Job drawing, mm, ordinate dimensions from the low corner. One solid piece. A direction names the side the tool comes from. Coordinates: 2 decimals unless noted, no trailing zeros. Write each loop counter-clockwise with the first axis right and the second up, starting at its lowest first coordinate (ties: lowest second). Pieces come first, ordered by that corner, then holes. Notation, with made-up numbers: (74.25, -38) - (103.25, -38) arc R19 ccw to (103.25, -22) - close; hole circle Ø10 at (46.25, 12.25). An arc over 180 degrees is marked (long way). Put each result on its own line as item: value. Start each with the question number.
1. Saw through at D-D, the plane y = 132.1. Write the cut outline in (x, z).
2. Which spindle directions (+Z, -Z, +X, -X, +Y, -Y) get a long thin tool onto all of the face, cutting with end or side? Do the marked faces 1 and 2. Say none if no direction does.
3. Drop flat-ended pins along their axis: P1, Ø3.5, axis at x = 8, y = 7.5, coming from the +Z side; P2, Ø1.2, axis at x = 133, y = 132, coming from the +Z side. Give the stop position or say it passes through.
4. Saw through at A-A, the plane x = 74. Write the cut outline in (y, z), plus the area to 3 significant figures.
5. Saw through at C-C, the plane z = 9. Write the cut outline in (x, y), plus the area to 3 significant figures.
6. Drill centre lines: L1, parallel to Y at x = 72.5, z = 8; L2, parallel to Y at x = 7.9, z = 17.75. Where is each one in solid material? Low to high. Write a range as from..to.
7. Pull direction X, two halves, no side cores. Call the marked faces 3, 4 and 5: released by +X, released by -X, zero draft, split by the parting line, or undercut.
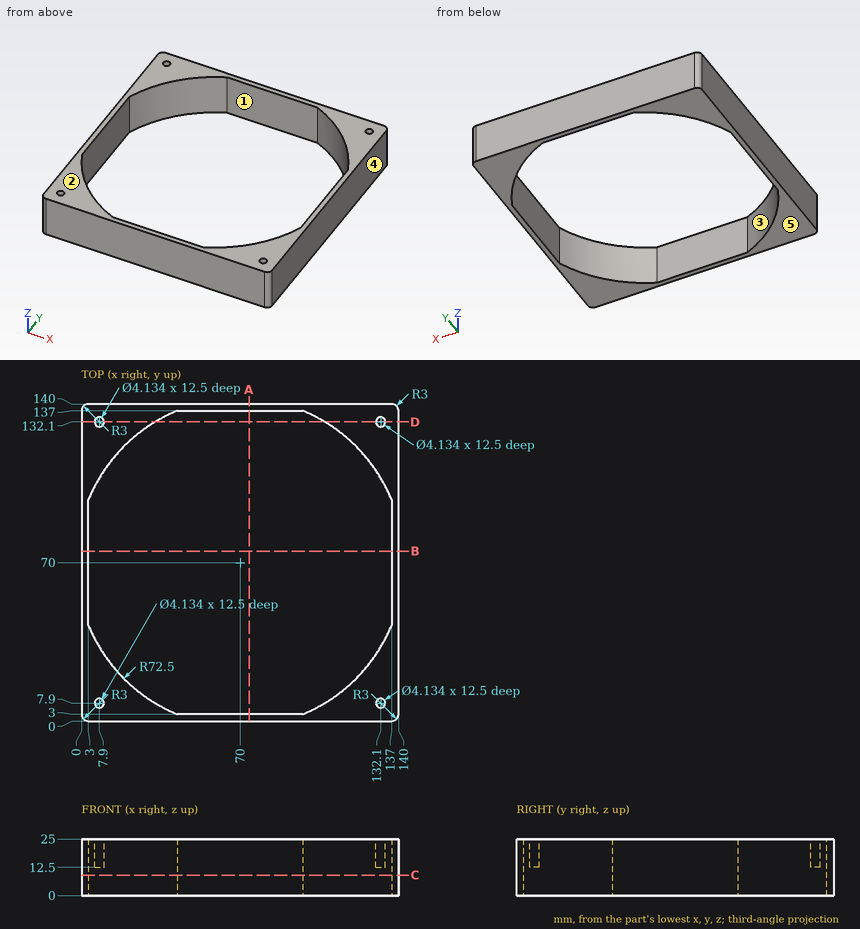
Final values:
1. outline: (0, 0) - (32.59, 0) - (32.59, 25) - (9.97, 25) - (9.97, 12.5) - (5.83, 12.5) - (5.83, 25) - (0, 25) - close; (107.41, 0) - (140, 0) - (140, 25) - (134.17, 25) - (134.17, 12.5) - (130.03, 12.5) - (130.03, 25) - (107.41, 25) - close
2. face 1: +Z, -Z
2. face 2: +Z, +X, -X, +Y, -Y
3. P1: stops at z = 25
3. P2: stops at z = 12.5
4. outline: (0, 0) - (3, 0) - (3, 25) - (0, 25) - close; (137, 0) - (140, 0) - (140, 25) - (137, 25) - close
4. area: 150 mm²
5. outline: (0, 3) arc R3 ccw to (3, 0) - (137, 0) arc R3 ccw to (140, 3) - (140, 137) arc R3 ccw to (137, 140) - (3, 140) arc R3 ccw to (0, 137) - close; hole (3, 42.3) arc R72.5 ccw to (42.3, 3) - (97.7, 3) arc R72.5 ccw to (137, 42.3) - (137, 97.7) arc R72.5 ccw to (97.7, 137) - (42.3, 137) arc R72.5 ccw to (3, 97.7) - close
5. area: 3,900 mm²
6. L1: y = 0..3, 137..140
6. L2: y = 0..5.83, 9.97..32.59, 107.41..130.03, 134.17..140
7. face 3: undercut
7. face 4: released by +X
7. face 5: zero draft
